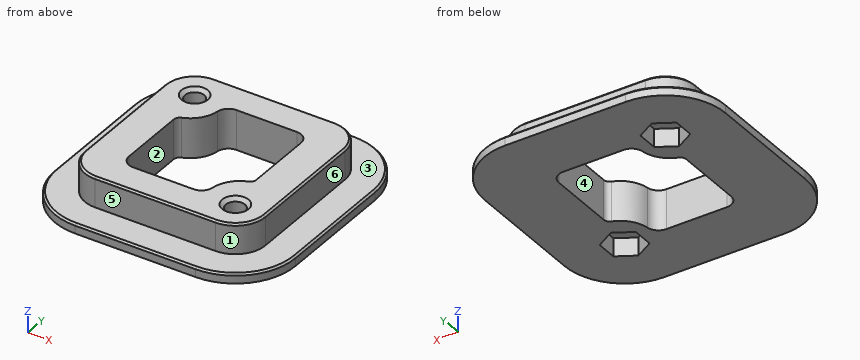
```python
from build123d import *

# Parameters (mm, degrees)
SKIZZE1_W          = 30
SKIZZE1_H          = 30
GRUNDK_RPER_DEPTH  = 5
VERRUNDUNG1_R      = 5
ABSATZ_DEPTH       = 1.6
SKIZZE3_R          = 1.6
M3_BOHRUNGEN_DEPTH = 30.044104393
M3_SCHSKANT_DEPTH  = 3
DURCHBRUCH_DEPTH   = 30.044104393
VERRUNDUNG2_R      = 5
VERRUNDUNG3_R      = 2
VERRUNDUNG4_R      = 1
FASE1_SIZE         = 0.3
FASE2_SIZE         = 0.6


with BuildPart() as part:
    # Skizze1 → Grundkörper (new body)
    with BuildSketch(Plane.XY):
        Rectangle(SKIZZE1_W, SKIZZE1_H)
    extrude(amount=GRUNDK_RPER_DEPTH)

    # Verrundung1
    verrundung1_edges = [part.edges().sort_by_distance(p)[0] for p in [
        (-15, 15, 2.5),
        (15, 15, 2.5),
        (15, -15, 2.5),
        (-15, -15, 2.5),
    ]]
    fillet(verrundung1_edges, radius=VERRUNDUNG1_R)

    # Skizze2 → Absatz (add)
    with BuildSketch(Plane(origin=(0, 0, 0), x_dir=(-1, 0, 0), z_dir=(0, 0, -1))):
        with BuildLine():
            Line((20, -10), (20, 10))
            ThreePointArc((20, 10), (17.071067812, 17.071067812), (10, 20))
            Line((10, 20), (-10, 20))
            ThreePointArc((-10, 20), (-17.071067812, 17.071067812), (-20, 10))
            Line((-20, 10), (-20, -10))
            ThreePointArc((-20, -10), (-17.071067812, -17.071067812), (-10, -20))
            Line((-10, -20), (10, -20))
            ThreePointArc((10, -20), (17.071067812, -17.071067812), (20, -10))
        make_face()
    extrude(amount=ABSATZ_DEPTH)

    # Skizze3 → M3 Bohrungen (cut, through all)
    with BuildSketch(Plane.XY.offset(5)):
        with Locations((-10, 10)):
            Circle(SKIZZE3_R)
        with Locations((10, -10)):
            Circle(SKIZZE3_R)
    extrude(amount=-M3_BOHRUNGEN_DEPTH, mode=Mode.SUBTRACT)

    # Skizze4 → M3 Schskant (cut)
    with BuildSketch(Plane(origin=(0, 0, -1.6), x_dir=(-1, 0, 0), z_dir=(0, 0, -1))):
        Polygon((10, 6.535898385), (13, 8.267949192), (13, 11.732050808), (10, 13.464101615), (7, 11.732050808), (7, 8.267949192), align=None)
        Polygon((-10, -6.535898385), (-13, -8.267949192), (-13, -11.732050808), (-10, -13.464101615), (-7, -11.732050808), (-7, -8.267949192), align=None)
    extrude(amount=-M3_SCHSKANT_DEPTH, mode=Mode.SUBTRACT)

    # Skizze5 → Durchbruch (cut, through all)
    with BuildSketch(Plane.XY.offset(5)):
        Polygon((5, 10), (-5, 10), (-5, 4), (-9, 4), (-9, -10), (-5, -10), (5, -10), (5, -4), (9, -4), (9, 10), align=None)
    extrude(amount=-DURCHBRUCH_DEPTH, mode=Mode.SUBTRACT)

    # Verrundung2
    # the kernel refuses this fillet: 5 mm, written as the material it takes off along each edge
    with BuildSketch(Plane(origin=(5, -4, 17.247448714), x_dir=(1.0, -1.5394352459447556e-12, 0), z_dir=(0, 0, -1)), Plane(origin=(-5, 4, 17.247448714), x_dir=(-1.0, 1.5605294834126232e-12, 0), z_dir=(0, 0, -1))) as verrundung2_piece_1:
        with BuildLine():
            CenterArc((5, 4.898979486), VERRUNDUNG2_R, 180, 78.463040967)
            Line((0, 4.898979486), (-0.1, 4.898979486))
            Line((-0.1, 4.898979486), (-0.1, 0))
            Line((-0.1, 0), (0, -0.1))
            ThreePointArc((0, -0.1), (2, -0.1), (3.98, -0.09797959))
            Line((3.98, -0.09797959), (4, 0))
        make_face()
    extrude(amount=31.094897428, mode=Mode.SUBTRACT)

    # Verrundung3
    verrundung3_edges = [part.edges().sort_by_distance(p)[0] for p in [
        (5, -10, 1.7),
        (-9, -10, 1.7),
        (-5, 10, 1.7),
        (9, 10, 1.7),
    ]]
    fillet(verrundung3_edges, radius=VERRUNDUNG3_R)

    # Verrundung4
    verrundung4_edges = [part.edges().sort_by_distance(p)[0] for p in [
        (-9, 4, 1.7),
        (9, -4, 1.7),
    ]]
    fillet(verrundung4_edges, radius=VERRUNDUNG4_R)

    # Fase1
    fase1_edges = [part.edges().sort_by_distance(p)[0] for p in [
        (-15, 0, 5),
        (0, 15, 5),
        (0, -15, 5),
        (15, 0, 5),
        (13.535533906, 13.535533906, 5),
        (13.535533906, -13.535533906, 5),
        (-13.535533906, -13.535533906, 5),
        (-13.535533906, 13.535533906, 5),
        (-17.071067812, -17.071067812, 0),
        (-20, 0, 0),
        (-17.071067812, 17.071067812, 0),
        (0, 20, 0),
        (17.071067812, 17.071067812, 0),
        (20, 0, 0),
        (17.071067812, -17.071067812, 0),
        (0, -20, 0),
    ]]
    chamfer(fase1_edges, length=FASE1_SIZE)

    # Fase2
    fase2_edges = [part.edges().sort_by_distance(p)[0] for p in [
        (-11.6, 10, 5),
        (8.4, -10, 5),
    ]]
    chamfer(fase2_edges, length=FASE2_SIZE)


solid = part.part
```
The model under review builds one solid part; all positions refer to its coordinate system, in mm. Face numbers are marked on the shaded views. A direction names the side the tool comes from. Round coordinates to 2 decimals unless told otherwise and drop trailing zeros. Order: outer loops, then holes, each group sorted by start corner. A loop starts at its lowest first (then second) coordinate and runs counter-clockwise, first axis right, second up.
Item 1: Add section C-C, the plane y = 5. State the section outline as (x, z) points, and give its area (3 significant figures).
Working result:
outline: (-20, -1.6) - (-6.87, -1.6) - (-6.87, 5) - (-14.7, 5) - (-15, 4.7) - (-15, 0) - (-19.7, 0) - (-20, -0.3) - close; (9, -1.6) - (20, -1.6) - (20, -0.3) - (19.7, 0) - (15, 0) - (15, 4.7) - (14.7, 5) - (9, 5) - close
area: 109 mm2
Item 2: To check wall thickness, follow probe 1 along Y at (x, z) = (-10, 2.7); probe 2 along Y at (x, z) = (10, 2.45); probe 3 along X at (y, z) = (5.5, 4.75). State the ranges of each line that lie inside material, in increasing order.
Working result:
probe 1: y = -15 to 8.4, 11.6 to 15
probe 2: y = -15 to -11.6, -8.4 to 15
probe 3: x = -14.95 to -6.33, 9 to 14.95
Item 3: Add section A-A, the plane y = -2.5. State the section outline as (x, z) points.
Working result:
outline: (-20, -1.6) - (-9, -1.6) - (-9, 5) - (-14.7, 5) - (-15, 4.7) - (-15, 0) - (-19.7, 0) - (-20, -0.3) - close; (9, -1.6) - (20, -1.6) - (20, -0.3) - (19.7, 0) - (15, 0) - (15, 4.7) - (14.7, 5) - (9, 5) - close
Item 4: Add section B-B, the plane z = 2.25. Count the separate pieces of the cut face and the enclosed holes in it, and give its area (3 significant figures).
Working result:
separate pieces: 1
enclosed holes: 3
area: 544 mm2
Item 5: Machinability: for the marked faces 1, 2 and 3, which of the approach directions +Z, -Z, +X, -X, +Y, -Y give a long, thin tool a straight path to every point of the face, cutting with its end or side? Answer none if there is none.
Working result:
face 1: +Z, +X, -Y
face 2: +Z, -Z
face 3: +Z
Item 6: Draft analysis for pull direction Y (two halves, no side actions). For the marked faces 4, 5 and 6, state which applies: released by +Y, released by -Y, zero draft, split by the parting line, or undercut.
Working result:
face 4: undercut
face 5: released by -Y
face 6: zero draft
Item 7: For pin 1 (1.8 mm diameter, centred on x = -9, y = 9, fed in from -Z); pin 2 (2 mm diameter, centred on x = -0.5, z = 3, fed in from -Y); pin 3 (1.5 mm diameter, centred on y = 10, z = 0, fed in from -X); pin 4 (1.4 mm diameter, centred on y = 2, z = 3.5, fed in from -X), all flat-tipped, find the tip position at first contact; note any pin that passes through.
Working result:
pin 1: stops at z = 1.4
pin 2: stops at y = -15
pin 3: stops at x = -20
pin 4: stops at x = -15
